```python
from build123d import *

# Parameters (mm, degrees)
SKETCH1_R           = 5
BOSS_EXTRUDE1_DEPTH = 7


with BuildPart() as part:
    # Sketch1 → Boss-Extrude1 (new body)
    with BuildSketch(Plane(origin=(0, 0, 0), x_dir=(1, 0, 0), z_dir=(0, 1, 0))):
        with BuildLine():
            Line((37.5, -4.5), (37.5, 4.5))
            Line((37.5, 4.5), (34.5, 7.5))
            Line((34.5, 7.5), (13.183654114, 7.5))
            ThreePointArc((13.183654114, 7.5), (7.556521898, 7.89778563), (2.041309299, 9.083230849))
            Line((2.041309299, 9.083230849), (-16.311620694, 14.406288432))
            ThreePointArc((-16.311620694, 14.406288432), (-35.49, 0), (-16.311620694, -14.406288432))
            Line((-16.311620694, -14.406288432), (2.041309299, -9.083230849))
            ThreePointArc((2.041309299, -9.083230849), (7.556521898, -7.89778563), (13.183654114, -7.5))
            Line((13.183654114, -7.5), (34.5, -7.5))
            Line((34.5, -7.5), (37.5, -4.5))
        make_face()
        with Locations((-20.49, 0)):
            Circle(SKETCH1_R, mode=Mode.SUBTRACT)
    extrude(amount=BOSS_EXTRUDE1_DEPTH)


solid = part.part
```
Design review of the part built by this model. Coordinates are the model's own, in mm. A direction names the side the tool comes from. Give positions to 0.01 mm unless a question says otherwise; leave off trailing zeros. Order: outer loops, then holes, each group sorted by start corner. A loop starts at its lowest first (then second) coordinate and runs counter-clockwise, first axis right, second up. Notation, with made-up numbers: (33, 0) -> (38, 0) arc R33 cw to (38, 38) -> close; hole circle Ø9 at (4, 1.25). An arc over 180 degrees is marked (long way). Write item = value, one per line. Start each with the question number.
(1) We need section A-A on x = -20.49. Write out the cut boundary in (y, z), plus the area to 3 significant figures.
(2) To check wall thickness, follow line 1 along Z through (x, y) = (-20.49, 3); line 2 along Z through (x, y) = (33.5, 4.25); line 3 along Z through (x, y) = (-23, 2.75). State the ranges of each line that lie inside material, in increasing order.
(3) For pin 1 (3.5 mm diameter, centred on x = 27.5, y = 3.5, fed in from +Z); pin 2 (1 mm diameter, centred on x = 2, y = 6, fed in from +Z); pin 3 (1.5 mm diameter, centred on y = 5.5, z = 6, fed in from +X), all flat-tipped, find the tip position at first contact; note any pin that passes through.
(4) We need section C-C on z = -3. Write out the cut boundary in (x, y).
(5) Mouldability with a two-part tool opening along Z and no side actions: class faces 4 (the face through (-25.485, 3.451, -0.22)), 5 (the face through (-7.01, 3.45, -11.71)), 6 (the face through (0, 0, 0)), 7 (the face through (-7.26, 3.45, 11.78)) as +Z half, -Z half, draft (parallel to the pull), parting line (faces both ways), or undercut.
(6) We need section D-D on x = 17.5. Write out the cut boundary in (y, z), plus the area to 3 significant figures.
(7) For faces 1 (the face through (24, 3, 7.5)), 2 (the face through (-35.485, 3.451, -0.389)), 3 (the face through (24, 3, -7.5)), list the 3-axis set-ups (+Z, -Z, +X, -X, +Y, -Y) from which the entire face can be reached by the end or side of a thin tool; tool diameter is ignored.
(8) We need section B-B on y = 2. Write out the cut boundary in (x, z).
Numbers:
q1.outline = (0, -15) -> (7, -15) -> (7, -5) -> (0, -5) -> close; (0, 5) -> (7, 5) -> (7, 15) -> (0, 15) -> close
q1.area = 140 mm^2
q2.line_1 = -15 to -5, 5 to 15
q2.line_2 = -7.5 to 7.5
q2.line_3 = -14.79 to -4.32, 4.32 to 14.79
q3.pin_1 = 7.5
q3.pin_2 = 9.24
q3.pin_3 = 36.75
q4.outline = (-35.19, 0) -> (-24.49, 0) -> (-24.49, 7) -> (-35.19, 7) -> close; (-16.49, 0) -> (37.5, 0) -> (37.5, 7) -> (-16.49, 7) -> close
q5.face_4 = undercut
q5.face_5 = -Z half
q5.face_6 = draft
q5.face_7 = +Z half
q6.outline = (0, -7.5) -> (7, -7.5) -> (7, 7.5) -> (0, 7.5) -> close
q6.area = 105 mm^2
q7.face_1 = +Z, +X, +Y, -Y
q7.face_2 = +Y, -Y
q7.face_3 = -Z, +X, +Y, -Y
q8.outline = (-16.31, -14.41) -> (2.04, -9.08) arc R40 cw to (13.18, -7.5) -> (34.5, -7.5) -> (37.5, -4.5) -> (37.5, 4.5) -> (34.5, 7.5) -> (13.18, 7.5) arc R40 cw to (2.04, 9.08) -> (-16.31, 14.41) arc R15 ccw (long way) to start; hole circle Ø10 at (-20.49, 0)
